Source: CAD feature listing. Evaluate the final solid. Frame: model axes, mm. Face numbers are marked on the shaded views. A direction names the side the tool comes from. Give positions to 0.01 mm unless a question says otherwise; leave off trailing zeros. Order: outer loops, then holes, each group sorted by start corner. A loop starts at its lowest first (then second) coordinate and runs counter-clockwise, first axis right, second up. Notation, with made-up numbers: M -3,87 L 32,87 A18 cw 32,113 Z; hole C -7,85 d4. An arc over 180 degrees is marked long. Return JSON: item names as keys, results as strings.
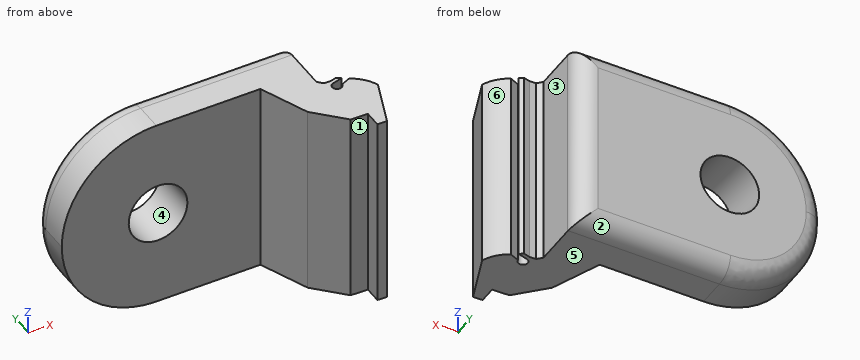
Autodesk Inventor part; units mm, degrees
ref_plane "YZ Plane" through (0, 0, 0) normal (1, 0, 0) x (0, 1, 0)
ref_plane "XZ Plane" through (0, 0, 0) normal (0, 1, 0) x (-1, 0, 0)
ref_plane "XY Plane" through (0, 0, 0) normal (0, 0, 1) x (1, 0, 0)
sketch "Sketch1" plane through (0, 0, 0) normal (0, 0, 1) x (1, 0, 0)
  line L0 (0, 0) -> (20.9872, 0.7329)
  line L1 (20.9872, 0.7329) -> (20.9872, -7.2671)
  line L2 (20.9872, -7.2671) -> (27.7872, -7.2671)
  line L3 (27.7872, -7.2671) -> (27.7872, -9.0671)
  line L4 (27.1872, -1.2671) -> (25.9872, -1.2671)
  line L5 (25.9872, -1.2671) -> (25.9872, 5.9105)
  line L6 (25.9872, 5.9105) -> (0, 5.003)
  line L7 (0, 5.003) -> (0, 0)
  line L8 (30.7063, -3.7945) -> (28.7872, -9.0671)
  line L9 (28.7872, -9.0671) -> (27.7872, -9.0671)
  line L10 (27.1872, -1.2671) -> (27.8551, -1.0596)
  line L11 (27.8551, -1.0596) -> (28.2648, -1.3511)
  line L12 (28.2648, -1.3511) -> (27.2091, -1.6792)
  arc A0 (30.7063, -3.7945) -> (28.8522, -1.7285) centre (26.9872, -5.2671) ccw
  arc A1 (27.2091, -1.6792) -> (27.8551, -2.2058) centre (27.3575, -2.1566) ccw
  line L13 (27.8551, -2.2058) -> (28.8522, -1.7285)
  point P0 (30.7872, -1.2671)
  dimension "d0" = 21
  dimension "d1" = 5
  dimension "d2" = 5
  dimension "d4" = 1.8
  dimension "d5" = 6
  dimension "d6" = 1.8
  dimension "d31" = 88
  dimension "d32" = 8
  dimension "d35" = 110
  dimension "d36" = 1
  dimension "d38" = 6
  dimension "d40" = 0.4
  dimension "d41" = 4
  dimension "d42" = 2
  dimension "d44" = 1.2
  dimension "d45" = 1
extrude "Extrusion1" add sketch "Sketch1" along normal blind 20
fillet "Fillet1" [suppressed]
fillet "Fillet2" radius 10 2 edges at (0, 2.5015, 0) (0, 2.5015, 20)
sketch "Sketch2" plane through (10, 5.3523, 10) normal (-0.0349, 0.9994, 0) x (0, 0, -1)
  circle A0 centre (0, 0) radius 3.1
  ellipse E0 centre (0, 0) end of major axis (0, 10.0061) minor radius 10 (10, 0) -> (-10, 0) ccw
  line L0 (-10, 0) -> (-10, -15.997)
  point P0 (10, 10.1807)
  dimension "d16" = 6.2
  dimension "d33" = 10
  dimension "d34" = 0
extrude "Extrusion2" cut sketch "Sketch2" against normal blind 10
fillet "Fillet3" radius 2 4 edges at (17.9934, 5.6314, 0) (2.9288, 5.1053, 2.9288) (17.9934, 5.6314, 20) (25.9872, 5.9105, 10)
chamfer "Chamfer2" distance 5 angle 45 1 edges at (20.9872, -7.2671, 10)
chamfer "Chamfer3" distance 3 angle 45 1 edges at (20.9872, -2.2671, 10)
chamfer "Chamfer4" distance 0.5 angle 45 1 edges at (25.9872, -1.2671, 10)
properties part number "PiedClip"
1. Draft query along X for the marked faces 4, 5 and 6. Return one class per face: pulls with the +X half, pulls with the -X half, needs draft (parallel to the pull), parting line crosses it, or undercut.
Evaluation:
{"face 4": "undercut", "face 5": "needs draft", "face 6": "pulls with the +X half"}
2. Section query A-A (y = -3). Return loops of the section in (x, z).
Evaluation:
{"outline": "M 22.53,0 L 30.28,0 L 30.28,20 L 22.53,20 Z"}
3. Ray query, probe 1 along Y at (x, z) = (26.5, 15); probe 2 along X at (y, z) = (3.5, 13.75); probe 3 along X at (y, z) = (-3.25, 9.75). Return the intervals inside material, ascending.
Evaluation:
{"probe 1": "y = -7.27 to -1.27", "probe 2": "x = 0.77 to 25.99", "probe 3": "x = 22.64 to 30.44"}
4. First-contact query: pin 1 (12 mm diameter, centred on x = 7.5, z = 14, fed in from -Y); pin 2 (0.6 mm diameter, centred on x = 27, z = 13.5, fed in from +Y); pin 3 (1.4 mm diameter, centred on y = 0.5, z = 7.5, fed in from +X); pin 4 (2 mm diameter, centred on x = 22, y = -6, fed in from +Z). Flat tips, straight axial feed; report the tip coordinate or a pass-through.
Evaluation:
{"pin 1": "stops at y = 0.05", "pin 2": "stops at y = -1.23", "pin 3": "stops at x = 25.99", "pin 4": "passes through"}
5. Set-up query: the marked faces 1, 2 and 3. Return all of +Z, -Z, +X, -X, +Y, -Y with unobstructed straight access to the full face (end or side cutting, diameter ignored); none if empty.
Evaluation:
{"face 1": "+Z, -Z, -X, -Y", "face 2": "-Z, -X, +Y", "face 3": "+Z, -Z, +X, +Y"}
